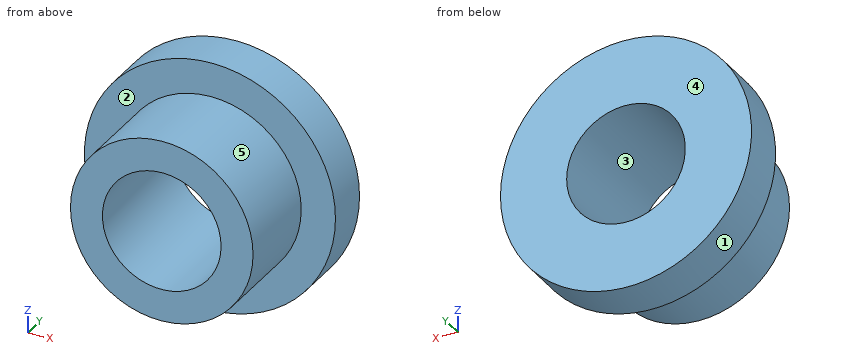
Autodesk Fusion 360 part; units mm, degrees
sketch "Sketch1" plane through (0, 0, 0) normal (0, 1, 0) x (1, 0, 0)
  circle A0 centre (0, 0) radius 4
  circle A1 centre (0, 0) radius 2.6
  dimension "d1" = 8
  dimension "d2" = 5.2
extrude "Extrude1" add sketch "Sketch1" against normal blind 6 makes body 1
sketch "Sketch2" plane through (0, 0, 0) normal (0, 1, 0) x (1, 0, 0)
  circle A0 centre (0, 0) radius 5.5
  circle A1 centre (0, 0) radius 4
  dimension "d5" = 11
  dimension "d6" = 8
extrude "Extrude2" add sketch "Sketch2" against normal blind 2 bodies 1
copy_body "Body->Comp1" bodies 1 removing the originals makes body 2 in component "Component"
component "Component" placed x (1, 0, 0) y (0, 1, 0) z (0, 0, 1) at (0, 0, 0)
equation "d2 = 8 mm - 2.8 mm"
Geometry: final body of the model. Coordinates: model frame, mm. Face numbers are marked on the shaded views. A direction names the side the tool comes from. Round coordinates to 2 decimals unless told otherwise and drop trailing zeros. Order: outer loops, then holes, each group sorted by start corner. A loop starts at its lowest first (then second) coordinate and runs counter-clockwise, first axis right, second up. Notation, with made-up numbers: (71, -36.5) -> (97, -36.5) arc R32 cw to (97, -1.5) -> close; hole circle Ø9 at (53.25, 65). An arc over 180 degrees is marked (long way). Use one line per item in the form item = value. Start each with the question number.
1. Draft query along Z for the marked faces 3, 4 and 5. Return one class per face: pulls with the +Z half, pulls with the -Z half, needs draft (parallel to the pull), parting line crosses it, or undercut.
2. Cut plane B-B (x = 0). Return the cut outline in (y, z), then the cut area to 3 significant figures.
3. Cut plane C-C (y = -3.3). Return the cut outline in (x, z), then the cut area to 3 significant figures.
4. Cut plane D-D (x = 3.25). Return the cut outline in (y, z), then the cut area to 3 significant figures.
5. Reachability of the marked faces 1 and 2 from +Z, -Z, +X, -X, +Y, -Y: full face, straight path, thin tool, end or side. Return the list, or none.
6. Line query: probe 1 along X at (y, z) = (-4.6, 0); probe 2 along X at (y, z) = (-1.6, 0). Output: solid intervals per line, ascending.
7. Pin query (flat end, axial travel): pin 1 Ø4 at (x, z) = (0, 0) entering from +Y; pin 2 Ø3 at (x, y) = (4, -5) entering from +Z; pin 3 Ø2 at (y, z) = (-2.5, -2) entering from +X; pin 4 Ø2 at (x, y) = (-0.5, -3.5) entering from +Z. Return the tip coordinate at first contact, or that it passes through.
8. Cut plane A-A (z = 0). Return the cut outline in (x, y), then the cut area to 3 significant figures.
Solution:
q1.face_3 = undercut
q1.face_4 = needs draft
q1.face_5 = parting line crosses it
q2.outline = (-6, -4) -> (-2, -4) -> (-2, -5.5) -> (0, -5.5) -> (0, -2.6) -> (-6, -2.6) -> close; (-6, 2.6) -> (0, 2.6) -> (0, 5.5) -> (-2, 5.5) -> (-2, 4) -> (-6, 4) -> close
q2.area = 22.8 mm^2
q3.outline = circle Ø8 at (0, 0); hole circle Ø5.2 at (0, 0)
q3.area = 29.0 mm^2
q4.outline = (-6, -2.33) -> (-2, -2.33) -> (-2, -4.44) -> (0, -4.44) -> (0, 4.44) -> (-2, 4.44) -> (-2, 2.33) -> (-6, 2.33) -> close
q4.area = 36.4 mm^2
q5.face_1 = +Y, -Y
q5.face_2 = -Y
q6.probe_1 = -4 to -2.6, 2.6 to 4
q6.probe_2 = -5.5 to -2.6, 2.6 to 5.5
q7.pin_1 = through
q7.pin_2 = 3.12
q7.pin_3 = 5.38
q7.pin_4 = 4
q8.outline = (-5.5, -2) -> (-4, -2) -> (-4, -6) -> (-2.6, -6) -> (-2.6, 0) -> (-5.5, 0) -> close; (2.6, -6) -> (4, -6) -> (4, -2) -> (5.5, -2) -> (5.5, 0) -> (2.6, 0) -> close
q8.area = 22.8 mm^2
